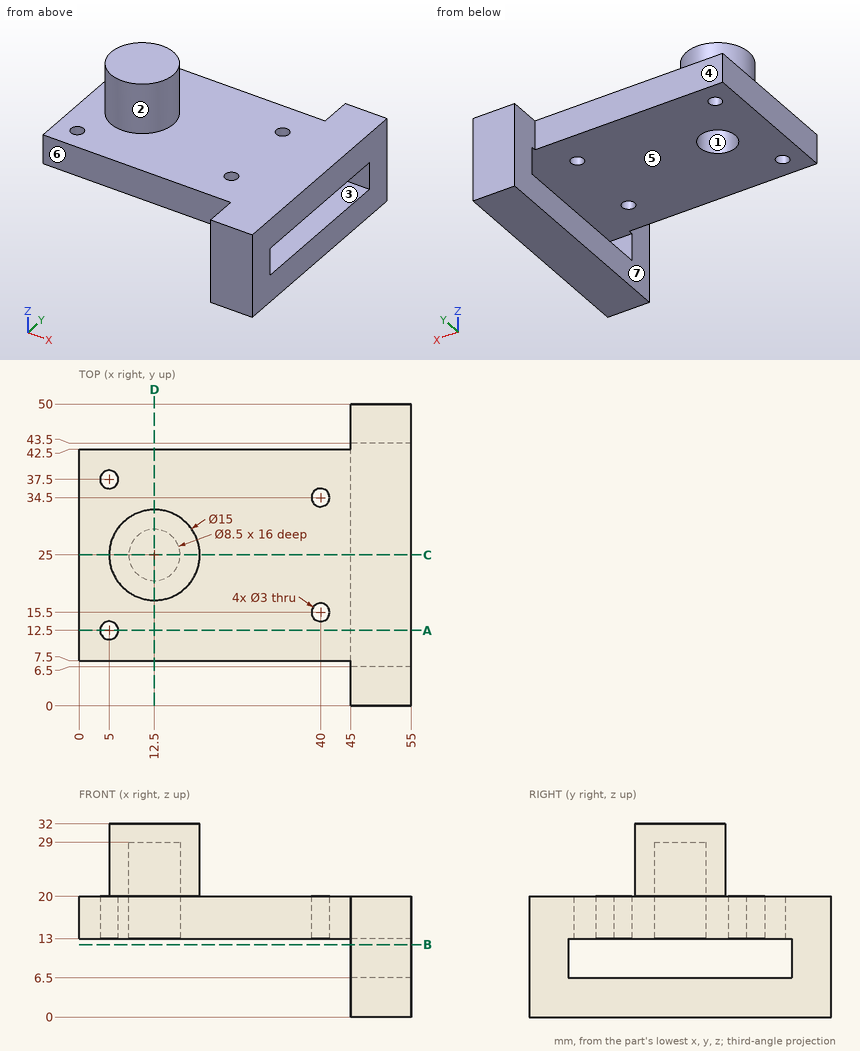
Source: three-view drawing plus pictorial views. Frame: mm from the lowest corner of the part. A direction names the side the tool comes from. Round coordinates to 2 decimals unless told otherwise and drop trailing zeros. Loops run counter-clockwise (first coordinate to the right, second up) from the corner with the lowest first, then second, coordinate; pieces in that order, holes last.
Q1. Section A-A on y = 12.5. Return loops of the section in (x, z), plus the area to 3 significant figures.
Q2. Section C-C on y = 25. Return loops of the section in (x, z).
Q3. Section D-D on x = 12.5. Return loops of the section in (y, z).
Q4. Section B-B on z = 12. Return loops of the section in (x, y), plus the area to 3 significant figures.
Q5. Pull-direction query (Y, two-part tool) for the marked faces 5, 6 and 7; classes: released by +Y, released by -Y, zero draft, split by the parting line, or undercut.
Q6. Access query for the marked faces 1, 2, 3 and 4. Directions: +Z, -Z, +X, -X, +Y, -Y. A direction counts if a zero-diameter tool reaches every point of the face in a straight line with its end or side. Return the directions, or none.
Q7. Pin query (flat end, axial travel): P1, Ø8, axis at x = 32, y = 9.5, coming from the -Z side; P2, Ø12, axis at x = 39, y = 23.5, coming from the +Z side; P3, Ø2.5, axis at x = 13.5, y = 25.5, coming from the -Z side. Return the tip coordinate at first contact, or that it passes through.
Q8. Material intervals for L1, parallel to Y at x = 5, z = 16; L2, parallel to Z at x = 47, y = 26; L3, parallel to Z at x = 17, y = 32, sorted ascending.
Evaluation:
1. outline: (0, 13) - (3.5, 13) - (3.5, 20) - (0, 20) - close; (6.5, 13) - (55, 13) - (55, 20) - (6.5, 20) - close; (45, 0) - (55, 0) - (55, 6.5) - (45, 6.5) - close
1. area: 429 mm2
2. outline: (0, 13) - (8.25, 13) - (8.25, 29) - (16.75, 29) - (16.75, 13) - (55, 13) - (55, 20) - (20, 20) - (20, 32) - (5, 32) - (5, 20) - (0, 20) - close; (45, 0) - (55, 0) - (55, 6.5) - (45, 6.5) - close
3. outline: (7.5, 13) - (20.75, 13) - (20.75, 29) - (29.25, 29) - (29.25, 13) - (42.5, 13) - (42.5, 20) - (32.5, 20) - (32.5, 32) - (17.5, 32) - (17.5, 20) - (7.5, 20) - close
4. outline: (45, 0) - (55, 0) - (55, 6.5) - (45, 6.5) - close; (45, 43.5) - (55, 43.5) - (55, 50) - (45, 50) - close
4. area: 130 mm2
5. face 5: undercut
5. face 6: released by -Y
5. face 7: zero draft
6. face 1: -Z
6. face 2: +Z
6. face 3: +X, -X
6. face 4: +Z, -Z, -X, +Y
7. P1: stops at z = 13
7. P2: stops at z = 20
7. P3: stops at z = 29
8. L1: y = 7.5 to 11, 14 to 36, 39 to 42.5
8. L2: z = 0 to 6.5, 13 to 20
8. L3: z = 13 to 20
